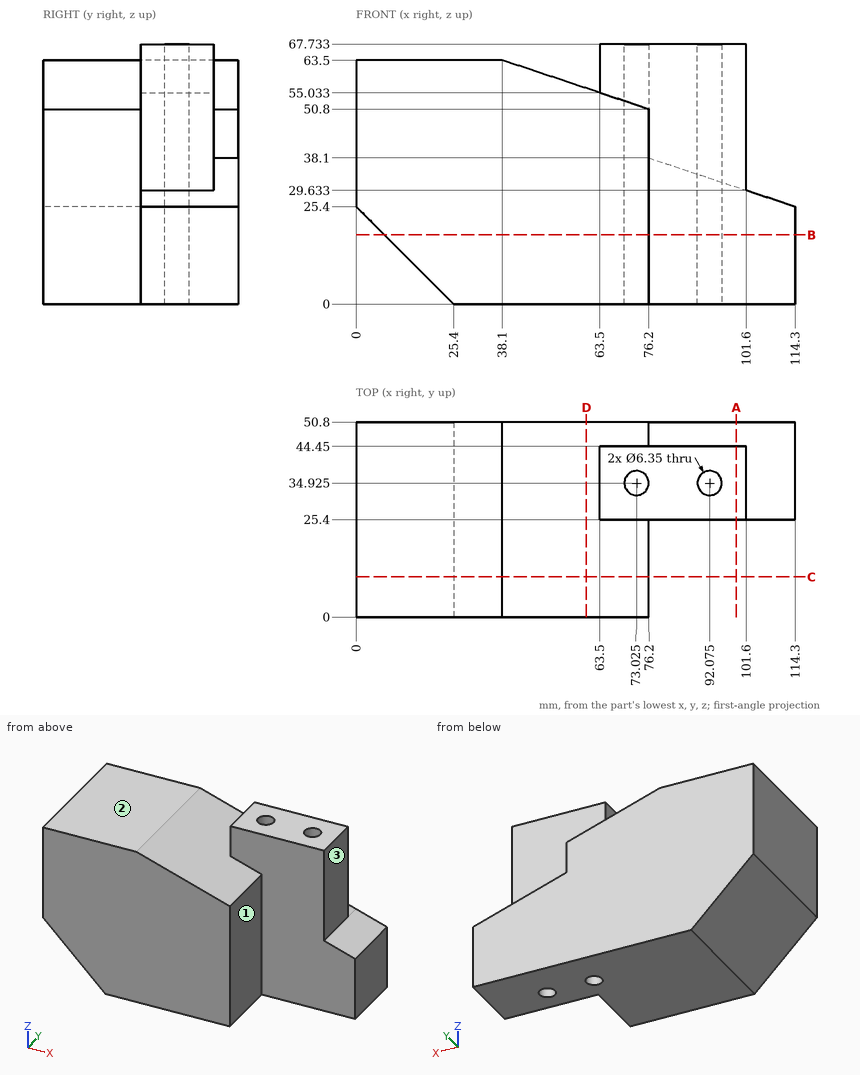
Job drawing, mm, ordinate dimensions from the low corner. One solid piece. A direction names the side the tool comes from. Coordinates: 2 decimals unless noted, no trailing zeros. Order: outer loops, then holes, each group sorted by start corner. A loop starts at its lowest first (then second) coordinate and runs counter-clockwise, first axis right, second up. Notation, with made-up numbers: M 63,-20 L 69,-20 A33 ccw 69,9 Z; hole C 89,-15 d1. An arc over 180 degrees is marked long. Return JSON: item names as keys, results as strings.
1. Saw through at B-B (z = 18). Give the number of separate pieces and of enclosed holes in the cut face, and give its area (3 significant figures).
Ans:
{"separate pieces": "1", "enclosed holes": "2", "area": "4,400 mm^2"}
2. Drill centre lines: probe 1 along Y at (x, z) = (102, 9.5); probe 2 along Y at (x, z) = (85.5, 36.5); probe 3 along Z at (x, y) = (33, 35). Where is each one in solid material? Low to high.
Ans:
{"probe 1": "25.4 to 50.8", "probe 2": "25.4 to 44.45", "probe 3": "0 to 63.5"}
3. Saw through at A-A (x = 99). Give the cut face in (y, z).
Ans:
{"outline": "M 25.4,0 L 50.8,0 L 50.8,30.5 L 44.45,30.5 L 44.45,67.73 L 25.4,67.73 Z"}
4. Flat gauge pins, fed straight in: pin 1 (7.5 mm diameter, centred on y = 16.5, z = 35.5, fed in from +X); pin 2 (4 mm diameter, centred on x = 73.025, y = 34.925, fed in from -Z); pin 3 (6 mm diameter, centred on y = 43.5, z = 59.5, fed in from +X); pin 4 (10 mm diameter, centred on x = 40, y = 18, fed in from +Z). Where does each tip first touch, or does it go through?
Ans:
{"pin 1": "x = 76.2", "pin 2": "through", "pin 3": "x = 101.6", "pin 4": "z = 63.5"}
5. Tool access for the marked faces 1, 2 and 3: list every direction of +Z, -Z, +X, -X, +Y, -Y with a clear straight run to the whole face (end or side of a thin tool).
Ans:
{"face 1": "+Z, -Z, +X, -Y", "face 2": "+Z, -X, +Y, -Y", "face 3": "+Z, +X, +Y, -Y"}
6. Saw through at D-D (x = 60). Give the cut face in (y, z).
Ans:
{"outline": "M 0,0 L 50.8,0 L 50.8,56.2 L 0,56.2 Z"}
7. Saw through at C-C (y = 10.5). Give the cut face in (x, z).
Ans:
{"outline": "M 0,25.4 L 25.4,0 L 76.2,0 L 76.2,50.8 L 38.1,63.5 L 0,63.5 Z"}
